The model under review builds one solid part; all positions refer to its coordinate system, in mm. A direction names the side the tool comes from. Coordinates: 2 decimals unless noted, no trailing zeros. Write each loop counter-clockwise with the first axis right and the second up, starting at its lowest first coordinate (ties: lowest second). Pieces come first, ordered by that corner, then holes. Notation, with made-up numbers: (34.5, 14) - (43.5, 14) arc R27 ccw to (43.5, 32) - close; hole circle Ø8 at (43.5, 69.5). An arc over 180 degrees is marked (long way). Answer as CSV lines item,"result". Start each with the question number.
```python
from build123d import *

# Parameters (mm, degrees)
SKETCH1_W           = 32
SKETCH1_H           = 32
BOSS_EXTRUDE1_DEPTH = 1
SKETCH2_R           = 1
CUT_EXTRUDE1_DEPTH  = 1
SKETCH3_R           = 5
BOSS_EXTRUDE2_DEPTH = 10
SKETCH4_W           = 10
SKETCH4_H           = 4.5
BOSS_EXTRUDE3_DEPTH = 6
SKETCH5_R           = 1.1
CUT_EXTRUDE2_DEPTH  = 2


with BuildPart() as part:
    # Sketch1 → Boss-Extrude1 (new body)
    with BuildSketch(Plane.XY):
        Rectangle(SKETCH1_W, SKETCH1_H)
    extrude(amount=BOSS_EXTRUDE1_DEPTH)

    # Sketch2 → Cut-Extrude1 (cut)
    with BuildSketch(Plane.XY.offset(1)):
        with Locations((-11, 11)):
            Circle(SKETCH2_R)
        with Locations((11, 11)):
            Circle(SKETCH2_R)
        with Locations((11, -11)):
            Circle(SKETCH2_R)
        with Locations((-11, -11)):
            Circle(SKETCH2_R)
    extrude(amount=-CUT_EXTRUDE1_DEPTH, mode=Mode.SUBTRACT)

    # Sketch3 → Boss-Extrude2 (add)
    with BuildSketch(Plane.XY.offset(1)):
        Circle(SKETCH3_R)
    extrude(amount=BOSS_EXTRUDE2_DEPTH)

    # Sketch4 → Boss-Extrude3 (add)
    with BuildSketch(Plane(origin=(0, 0, 0), x_dir=(-1, 0, 0), z_dir=(0, 0, -1))):
        with Locations((-3, -12.25)):
            Rectangle(SKETCH4_W, SKETCH4_H)
    extrude(amount=BOSS_EXTRUDE3_DEPTH)

    # Sketch5 → Cut-Extrude2 (cut)
    with BuildSketch(Plane.XY.offset(1)):
        with Locations((-14.2, 14.2)):
            Circle(SKETCH5_R)
        with Locations((14.2, 14.2)):
            Circle(SKETCH5_R)
        with Locations((14.2, -14.2)):
            Circle(SKETCH5_R)
        with Locations((-14.2, -14.2)):
            Circle(SKETCH5_R)
    extrude(amount=-CUT_EXTRUDE2_DEPTH, mode=Mode.SUBTRACT)


solid = part.part
```
(1) Add section C-C on y = -3.5. Give the boundary of the cut face in (x, z), then the cut area to 3 significant figures.
(2) Add section D-D on y = 10.5. Give the boundary of the cut face in (x, z), then the cut area to 3 significant figures.
(3) Wall thickness on line 1 (Y direction, x = -11, z = 0.4); line 2 (Y direction, x = 14.2, z = 0.55); line 3 (Z direction, x = -9, y = 2.5): over which ranges is each line inside the solid? List them lowest first.
(4) The part is to be moulded in two halves that separate along Y. For faces 5 (the flat face through (-2, -12, -3)), 6 (the flat face through (3, -14.5, -3)), 7 (the cylindrical face through (14.79, -13.27, 0.51)), say which applies: released by +Y, released by -Y, zero draft, split by the parting line, or undercut.
(5) Add section A-A on y = -11. Give the boundary of the cut face in (x, z).
(6) For pin 1 (8 mm diameter, centred on y = 5, z = 9, fed in from +X); pin 2 (2.5 mm diameter, centred on x = -11, y = 11, fed in from +Z); pin 3 (3.5 mm diameter, centred on x = 14.2, y = 14.2, fed in from -Z); pin 4 (1.8 mm diameter, centred on x = -11, y = -11, fed in from -Z), all flat-tipped, find the tip position at first contact; note any pin that passes through.
(7) Add section B-B on x = -11. Give the boundary of the cut face in (y, z).
(8) For faces 1 (the flat face through (0, 0, 11)), 2 (the cylindrical face through (-1.08, -4.88, 5.93)), 3 (the flat face through (8, -12, -3)), 4 (the flat face through (3, -10, -3)), list the 3-axis set-ups (+Z, -Z, +X, -X, +Y, -Y) from which the entire face can be reached by the end or side of a thin tool; tool diameter is ignored.
Reported:
1,outline,"(-16, 0) - (16, 0) - (16, 1) - (3.57, 1) - (3.57, 11) - (-3.57, 11) - (-3.57, 1) - (-16, 1) - close"
1,area,"103 mm²"
2,outline,"(-16, 0) - (-11.87, 0) - (-11.87, 1) - (-16, 1) - close; (-10.13, 0) - (10.13, 0) - (10.13, 1) - (-10.13, 1) - close; (11.87, 0) - (16, 0) - (16, 1) - (11.87, 1) - close"
2,area,"28.5 mm²"
3,line 1,"-16 to -12, -10 to 10, 12 to 16"
3,line 2,"-16 to -15.3, -13.1 to 13.1, 15.3 to 16"
3,line 3,"0 to 1"
4,face 5,"zero draft"
4,face 6,"released by -Y"
4,face 7,"undercut"
5,outline,"(-16, 0) - (-12, 0) - (-12, 1) - (-16, 1) - close; (-10, 0) - (-2, 0) - (-2, -6) - (8, -6) - (8, 0) - (10, 0) - (10, 1) - (-10, 1) - close; (12, 0) - (16, 0) - (16, 1) - (12, 1) - close"
6,pin 1,"x = 4.9"
6,pin 2,"z = 1"
6,pin 3,"z = 0"
6,pin 4,"through"
7,outline,"(-16, 0) - (-12, 0) - (-12, 1) - (-16, 1) - close; (-10, 0) - (10, 0) - (10, 1) - (-10, 1) - close; (12, 0) - (16, 0) - (16, 1) - (12, 1) - close"
8,face 1,"+Z, +X, -X, +Y, -Y"
8,face 2,"+Z"
8,face 3,"-Z, +X, +Y, -Y"
8,face 4,"-Z, +X, -X, +Y"
